```python
from build123d import *

# Parameters (mm, degrees)
SKETCH_281X300_25_R   = 1.6
SKETCH_281X300_25_R_2 = 15
SKETCH_281X300_25_R_3 = 2.15
SKETCH_281X300_25_R_4 = 2.2
SKETCH_281X300_25_W   = 73
SKETCH_281X300_25_H   = 40
F_4MM_DEPTH           = 4
FILLET_1_R            = 8


with BuildPart() as part:
    # Sketch 281x300__25 → 4mm (new body)
    with BuildSketch(Plane.XY):
        Polygon((-51, 150), (53, 150), (53, 100), (137.5, 100), (137.5, -100), (53, -100), (53, -150), (-51, -150), (-51, -100), (-135.5, -100), (-135.5, 100), (-51, 100), align=None)
        with Locations((84.5, -60)):
            Circle(SKETCH_281X300_25_R, mode=Mode.SUBTRACT)
        with Locations((114.5, -60)):
            Circle(SKETCH_281X300_25_R, mode=Mode.SUBTRACT)
        with Locations((84.5, 61)):
            Circle(SKETCH_281X300_25_R, mode=Mode.SUBTRACT)
        with Locations((1, 90.5)):
            Circle(SKETCH_281X300_25_R_2, mode=Mode.SUBTRACT)
        with Locations((1, 125)):
            Circle(SKETCH_281X300_25_R_3, mode=Mode.SUBTRACT)
        with Locations((-33.5, 90.5)):
            Circle(SKETCH_281X300_25_R_3, mode=Mode.SUBTRACT)
        with Locations((35.5, 90.5)):
            Circle(SKETCH_281X300_25_R_3, mode=Mode.SUBTRACT)
        with Locations((-44, 140)):
            Circle(SKETCH_281X300_25_R_3, mode=Mode.SUBTRACT)
        with Locations((114.5, 61)):
            Circle(SKETCH_281X300_25_R, mode=Mode.SUBTRACT)
        with Locations((1, 56)):
            Circle(SKETCH_281X300_25_R_3, mode=Mode.SUBTRACT)
        with Locations((26, -140)):
            Circle(SKETCH_281X300_25_R_4, mode=Mode.SUBTRACT)
        with Locations((-24, -140)):
            Circle(SKETCH_281X300_25_R_4, mode=Mode.SUBTRACT)
        with Locations((-24, -90)):
            Circle(SKETCH_281X300_25_R_4, mode=Mode.SUBTRACT)
        with Locations((26, -90)):
            Circle(SKETCH_281X300_25_R_4, mode=Mode.SUBTRACT)
        with Locations((1, 111.5)):
            Circle(SKETCH_281X300_25_R, mode=Mode.SUBTRACT)
        with Locations((84.5, -90)):
            Circle(SKETCH_281X300_25_R, mode=Mode.SUBTRACT)
        with Locations((84.5, 91)):
            Circle(SKETCH_281X300_25_R, mode=Mode.SUBTRACT)
        with Locations((114.5, 91)):
            Circle(SKETCH_281X300_25_R, mode=Mode.SUBTRACT)
        with Locations((114.5, -90)):
            Circle(SKETCH_281X300_25_R, mode=Mode.SUBTRACT)
        with Locations((118.5, 10)):
            Circle(SKETCH_281X300_25_R, mode=Mode.SUBTRACT)
        with Locations((118.5, -10)):
            Circle(SKETCH_281X300_25_R, mode=Mode.SUBTRACT)
        with Locations((-120.5, 10)):
            Circle(SKETCH_281X300_25_R, mode=Mode.SUBTRACT)
        with Locations((-120.5, -10)):
            Circle(SKETCH_281X300_25_R, mode=Mode.SUBTRACT)
        with Locations((-115.5, -91)):
            Circle(SKETCH_281X300_25_R, mode=Mode.SUBTRACT)
        with Locations((-85.5, -91)):
            Circle(SKETCH_281X300_25_R, mode=Mode.SUBTRACT)
        with Locations((-115.5, 91)):
            Circle(SKETCH_281X300_25_R, mode=Mode.SUBTRACT)
        with Locations((-85.5, 91)):
            Circle(SKETCH_281X300_25_R, mode=Mode.SUBTRACT)
        with Locations((-85.5, 61)):
            Circle(SKETCH_281X300_25_R, mode=Mode.SUBTRACT)
        with Locations((-115.5, 61)):
            Circle(SKETCH_281X300_25_R, mode=Mode.SUBTRACT)
        with Locations((-85.5, -61)):
            Circle(SKETCH_281X300_25_R, mode=Mode.SUBTRACT)
        with Locations((-115.5, -61)):
            Circle(SKETCH_281X300_25_R, mode=Mode.SUBTRACT)
        with Locations((118.5, 43)):
            Circle(SKETCH_281X300_25_R, mode=Mode.SUBTRACT)
        with Locations((118.5, -42)):
            Circle(SKETCH_281X300_25_R, mode=Mode.SUBTRACT)
        with Locations((-120.5, 43)):
            Circle(SKETCH_281X300_25_R, mode=Mode.SUBTRACT)
        with Locations((46, 140)):
            Circle(SKETCH_281X300_25_R_3, mode=Mode.SUBTRACT)
        with Locations((-44, -140)):
            Circle(SKETCH_281X300_25_R_3, mode=Mode.SUBTRACT)
        with Locations((46, -140)):
            Circle(SKETCH_281X300_25_R_3, mode=Mode.SUBTRACT)
        with Locations((19.186533479, 101)):
            Circle(SKETCH_281X300_25_R, mode=Mode.SUBTRACT)
        with Locations((19.186533479, 80)):
            Circle(SKETCH_281X300_25_R, mode=Mode.SUBTRACT)
        with Locations((1, 69.5)):
            Circle(SKETCH_281X300_25_R, mode=Mode.SUBTRACT)
        with Locations((-17.186533479, 80)):
            Circle(SKETCH_281X300_25_R, mode=Mode.SUBTRACT)
        with Locations((-17.186533479, 101)):
            Circle(SKETCH_281X300_25_R, mode=Mode.SUBTRACT)
        with Locations((-120.5, -43)):
            Circle(SKETCH_281X300_25_R, mode=Mode.SUBTRACT)
        with BuildLine():
            Line((68.5, -50), (68.5, -36))
            ThreePointArc((68.5, -36), (61, -28.5), (53.5, -36))
            Line((53.5, -36), (53.5, -50))
            ThreePointArc((53.5, -50), (61, -57.5), (68.5, -50))
        make_face(mode=Mode.SUBTRACT)
        with BuildLine():
            Line((-95.5, -10), (-75.5, -10))
            ThreePointArc((-75.5, -10), (-65.5, 0), (-75.5, 10))
            Line((-75.5, 10), (-95.5, 10))
            ThreePointArc((-95.5, 10), (-105.5, 0), (-95.5, -10))
        make_face(mode=Mode.SUBTRACT)
        with Locations((1, -115)):
            Rectangle(SKETCH_281X300_25_W, SKETCH_281X300_25_H, mode=Mode.SUBTRACT)
        with BuildLine():
            Line((53.5, 29), (53.5, 15))
            ThreePointArc((53.5, 15), (61, 7.5), (68.5, 15))
            Line((68.5, 15), (68.5, 29))
            ThreePointArc((68.5, 29), (61, 36.5), (53.5, 29))
        make_face(mode=Mode.SUBTRACT)
    extrude(amount=F_4MM_DEPTH)

    # Fillet 1
    fillet_1_edges = [part.edges().sort_by_distance(p)[0] for p in [
        (53, -150, 2),
        (-51, -150, 2),
        (-51, -100, 2),
        (-135.5, -100, 2),
        (-135.5, 100, 2),
        (-51, 100, 2),
        (-51, 150, 2),
        (53, 150, 2),
        (53, 100, 2),
        (137.5, 100, 2),
        (137.5, -100, 2),
        (53, -100, 2),
        (-35.5, -95, 2),
        (-35.5, -135, 2),
        (37.5, -135, 2),
        (37.5, -95, 2),
    ]]
    fillet(fillet_1_edges, radius=FILLET_1_R)


solid = part.part
```
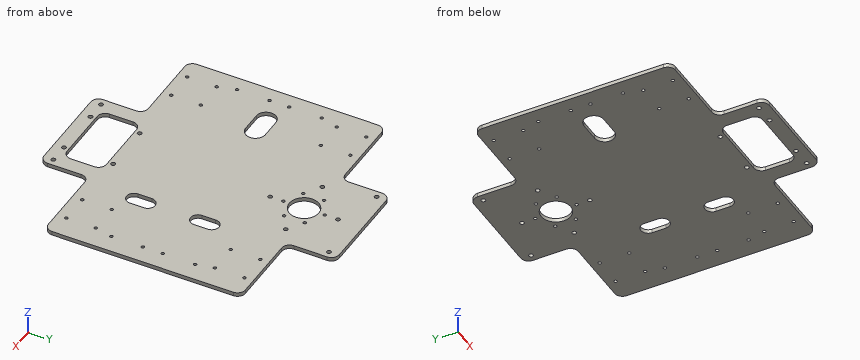
Read the model definition and answer for the solid it produces. Units are mm, in the model's axes. Give positions to 0.01 mm unless a question says otherwise; leave off trailing zeros. Write each loop counter-clockwise with the first axis right and the second up, starting at its lowest first coordinate (ties: lowest second). Pieces come first, ordered by that corner, then holes. Notation, with made-up numbers: (23, -38.75) -> (62, -38.75) arc R21 ccw to (62, -27.75) -> close; hole circle Ø2 at (-40, 35). An arc over 180 degrees is marked (long way). Answer in a Markdown table with one row per item.
1) Each of these flat-tipped pins is pushed along its axis until it touches: pin 1 Ø12 at (x, y) = (-103, 37.5) entering from -Z; pin 2 Ø3 at (x, y) = (1, 111.5) entering from -Z; pin 3 Ø1.2 at (y, z) = (131, 2.5) entering from -X; pin 4 Ø1 at (x, z) = (-60.5, 1.5) entering from +Y. Where does it stop, or does it pass through?
Results list:
| item | result |
|---|---|
| pin 1 | z = 0 |
| pin 2 | through |
| pin 3 | x = -51 |
| pin 4 | y = 100 |
2) Section B-B on z = 2 is taken. Count the separate pieces of the cut face and the enclosed holes in it, plus the area to 3 significant figures.
Results list:
| item | result |
|---|---|
| separate pieces | 1 |
| enclosed holes | 47 |
| area | 59,500 mm^2 |
3) Section A-A on y = 0 is taken. Give the vertices of the cut face in (x, z), plus the area to 3 significant figures.
Results list:
| item | result |
|---|---|
| outline | (-135.5, 0) -> (-105.5, 0) -> (-105.5, 4) -> (-135.5, 4) -> close; (-65.5, 0) -> (137.5, 0) -> (137.5, 4) -> (-65.5, 4) -> close |
| area | 932 mm^2 |
4) Straight lines are drawn through the part: line 1 (Y direction, x = -120.5, z = 0.8); line 2 (Y direction, x = 84.5, z = 3.2); line 3 (X direction, y = 80, z = 2.35). For each, find the intervals that lie inside material, in ascending order. Write a range as [from, to].
Results list:
| item | result |
|---|---|
| line 1 | [-100, -44.6], [-41.4, -11.6], [-8.4, 8.4], [11.6, 41.4], [44.6, 100] |
| line 2 | [-100, -91.6], [-88.4, -61.6], [-58.4, 59.4], [62.6, 89.4], [92.6, 100] |
| line 3 | [-135.5, -18.79], [-15.59, -9.71], [11.71, 17.59], [20.79, 137.5] |
